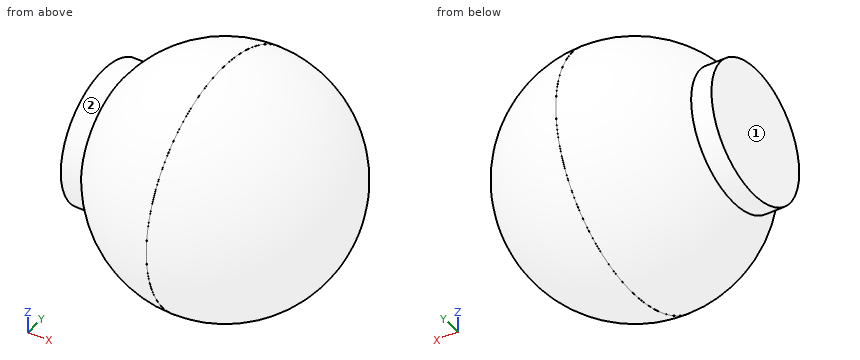
from build123d import *

# Parameters (mm, degrees)
F0_R     = 57.15
F1_DEPTH = 57.15
F2_R     = 57.15
F3_DEPTH = 57.15
F4_R     = 57.14999
F5_R     = 57.14999
F6_R     = 31.75
F7_DEPTH = 57.15


# Not quite as in the source:
# - a fillet or chamfer is up to 0.001 mm smaller than in the source, because OpenCascade refuses the exact size


with BuildPart() as f1:
    # F0 (on Right) → F1 (new body)
    with BuildSketch(Plane.YZ):
        Circle(F0_R)
    extrude(amount=F1_DEPTH)

    # F2 (on face) → F3 (join)
    with BuildSketch(Plane(origin=(0, 0, 0), x_dir=(0, -1, 0), z_dir=(-1, 0, 0))):
        Circle(F2_R)
    extrude(amount=F3_DEPTH)

    # F4 (radius 57.15 in the source; OpenCascade refuses exactly that, so slightly less here)
    f4_edges = [f1.edges().sort_by_distance(p)[0] for p in [
        (-57.15, 57.15, 0),
    ]]
    fillet(f4_edges, radius=F4_R)

    # F5 (radius 57.15 in the source; OpenCascade refuses exactly that, so slightly less here)
    f5_edges = [f1.edges().sort_by_distance(p)[0] for p in [
        (57.15, -57.15, 0),
    ]]
    fillet(f5_edges, radius=F5_R)

    # F6 (on face) → F7 (join)
    with BuildSketch(Plane(origin=(0, 0, 0), x_dir=(0, -1, 0), z_dir=(-1, 0, 0))):
        Circle(F6_R)
    extrude(amount=F7_DEPTH)


solid = f1.part
Check sheet for the modelled part. Datum: model origin and axes. Units: mm. Face numbers are marked on the shaded views. A direction names the side the tool comes from. Round coordinates to 2 decimals unless told otherwise and drop trailing zeros.
Q1. Depth check by flat-ended pin: P1, Ø1.5, axis at x = 15, z = -34, coming from the +Y side; P2, Ø3, axis at x = -16.5, y = 15.5, coming from the -Z side; P3, Ø2, axis at x = 11, z = 33.5, coming from the -Y side. Enter the tip coordinate at first touch or a pass-through.
Filled sheet:
P1: stops at y = 44.05
P2: stops at z = -53.1
P3: stops at y = -45.74
Q2. Set-up check for the marked faces 1 and 2: record each of +Z, -Z, +X, -X, +Y, -Y from which the full face is reachable in a straight line by a thin tool's end or side.
Filled sheet:
face 1: +Z, -Z, -X, +Y, -Y
face 2: -X
Q3. Scan lines: L1, parallel to Z at x = 20.5, y = -30; L2, parallel to Y at x = 47, z = 4.5. Record each from-to range of solid material in increasing order.
Filled sheet:
L1: z = -44.11 to 44.11
L2: y = -32.2 to 32.2
